Source: CAD feature listing. Evaluate the final solid. Frame: model axes, mm. Face numbers are marked on the shaded views. Round coordinates to 2 decimals unless told otherwise and drop trailing zeros. Order: outer loops, then holes, each group sorted by start corner. A loop starts at its lowest first (then second) coordinate and runs counter-clockwise, first axis right, second up. Notation, with made-up numbers: (-15, 23) - (40, 23) arc R21 cw to (40, 27) - close; hole circle Ø4 at (69, 4). An arc over 180 degrees is marked (long way). Use one line per item in the form item = value. Start each with the question number.
Q1. Draft query along Y for the marked faces 1, 2 and 3. Return one class per face: released by +Y, released by -Y, zero draft, split by the parting line, or undercut.
Q2. Cut plane A-A, the plane x = 36. Return the cut outline in (y, z), and give its area (3 significant figures).
Q3. Cut plane B-B, the plane z = -509. Return the cut outline in (x, y).
Q4. Cut plane C-C, the plane y = -495. Return the cut outline in (x, z).
Q5. Ray query, line 1 (Y direction, x = 0, z = -489.5); line 2 (X direction, y = -260.5, z = 6); line 3 (Z direction, x = -6.5, y = -305.5). Return the intervals inside material, ascending. Write a range as [from, to].
Q6. Pin query (flat end, axial travel): pin 1 Ø2 at (x, z) = (-45.5, 0) entering from +Y; pin 2 Ø6 at (x, y) = (22.5, -1083) entering from +Z; pin 3 Ø5 at (y, z) = (-750.5, 10) entering from -X. Return the tip coordinate at first contact, or that it passes through.
Q7. Cut plane D-D, the plane x = -101. Return the cut outline in (y, z), and give its area (3 significant figures).
from build123d import *

# Parameters (mm, degrees)
F0_R     = 150
F0_R_2   = 148
F3_DEPTH = 150
F4_R     = 200
F5_DEPTH = 1350.0010001


with BuildPart() as f2:
    # F2: sweep along a path in F1
    with BuildLine(Plane.YZ) as f2_path:
        Line((0, 0), (-800, 0))
        ThreePointArc((-800, 0), (-1082.8427124746, -117.1572875254), (-1200, -400))
        Line((-1200, -400), (-1200, -565))
    # F0 (on Front) → F2 (sweep)
    with BuildSketch(Plane.XZ):
        Circle(F0_R)
        Circle(F0_R_2, mode=Mode.SUBTRACT)
    sweep(path=f2_path.line)

    # F1 (on Right) → F3 (cut, symmetric)
    with BuildSketch(Plane.YZ):
        with BuildLine():
            ThreePointArc((-150, 0), (0, -150), (150, 0))
            ThreePointArc((150, 0), (0, 150), (-150, 0))
        make_face()
    extrude(amount=F3_DEPTH, both=True, mode=Mode.SUBTRACT)

    # F4 (on Front) → F5 (cut, through all)
    with BuildSketch(Plane.XZ):
        with Locations((0, -7129.1327476501)):
            Circle(F4_R)
    extrude(amount=F5_DEPTH, mode=Mode.SUBTRACT)


solid = f2.part
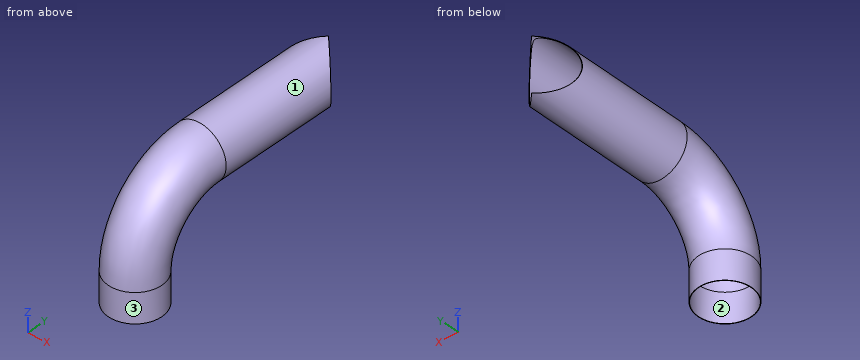
Completed:
q1.face_1 = zero draft
q1.face_2 = undercut
q1.face_3 = split by the parting line
q2.outline = (-1345.62, -565) - (-1343.55, -565) - (-1343.55, -400) arc R543.55 cw to (-800, 143.55) - (-43.5, 143.55) arc R150 cw to (-36, 145.62) - (-800, 145.62) arc R545.62 ccw to (-1345.62, -400) - close; (-1056.45, -565) - (-1054.38, -565) - (-1054.38, -400) arc R254.38 cw to (-800, -145.62) - (-36, -145.62) arc R150 cw to (-43.5, -143.55) - (-800, -143.55) arc R256.45 ccw to (-1056.45, -400) - close
q2.area = 6,400 mm2
q3.outline = circle Ø300 at (0, -1200); hole circle Ø296 at (0, -1200)
q4.outline = circle Ø300 at (0, 0); hole circle Ø296 at (0, 0)
q5.line_1 = [-1350, -1348], [-1052, -1050]
q5.line_2 = [-149.88, -147.88], [147.88, 149.88]
q5.line_3 = [-149.86, -147.86], [147.86, 149.86]
q6.pin_1 = -1162.8
q6.pin_2 = 71.49
q6.pin_3 = -149.81
q7.outline = (-1310.9, -565) - (-1308.18, -565) - (-1308.18, -400) arc R508.18 cw to (-800, 108.18) - (-103.91, 108.18) arc R150 cw to (-101, 110.9) - (-800, 110.9) arc R510.9 ccw to (-1310.9, -400) - close; (-1091.82, -565) - (-1089.1, -565) - (-1089.1, -400) arc R289.1 cw to (-800, -110.9) - (-101, -110.9) arc R150 cw to (-103.91, -108.18) - (-800, -108.18) arc R291.82 ccw to (-1091.82, -400) - close
q7.area = 8,110 mm2
